Can you work these out from the model? Positions are in its coordinate system, mm. A direction names the side the tool comes from. Give positions to 0.01 mm unless a question says otherwise; leave off trailing zeros. Loops run counter-clockwise (first coordinate to the right, second up) from the corner with the lowest first, then second, coordinate; pieces in that order, holes last. Notation, with made-up numbers: (-6, 58) - (43, 58) arc R3 cw to (43, 62) - close; hole circle Ø3 at (9.25, 2). An arc over 180 degrees is marked (long way). Answer in a Markdown table with one row per item.
Autodesk Inventor part; units mm, degrees
ref_plane "YZ Plane" through (0, 0, 0) normal (1, 0, 0) x (0, 1, 0)
ref_plane "XZ Plane" through (0, 0, 0) normal (0, 1, 0) x (-1, 0, 0)
ref_plane "XY Plane" through (0, 0, 0) normal (0, 0, 1) x (1, 0, 0)
sketch "スケッチ1" plane through (0, 0, 0) normal (0, 0, 1) x (1, 0, 0)
  line L0 (0, 0) -> (142, 0)
  line L1 (142, 0) -> (142, 80)
  line L2 (142, 80) -> (0, 80)
  line L3 (0, 80) -> (0, 0)
  dimension "d40" = 142
  dimension "d41" = 80
extrude "押し出し1" add sketch "スケッチ1" along normal blind 3.3
hole "穴5" at (4.5, 75.5, 3.3) direction (0, 0, -1) diameter 3.4 end through all
hole "穴6" at (137.5, 75.5, 3.3) direction (0, 0, -1) diameter 3.4 end through all
hole "穴7" at (137.5, 4.5, 3.3) direction (0, 0, -1) diameter 3.4 end through all
hole "穴8" at (4.5, 4.5, 3.3) direction (0, 0, -1) diameter 3.4 end through all
hole "穴9" at (130, 73, 3.3) direction (0, 0, -1) diameter 3.4 end through all
hole "穴10" at (130, 7, 3.3) direction (0, 0, -1) diameter 3.4 end through all
hole "穴13" at (41, 73, 3.3) direction (0, 0, -1) diameter 3.4 end through all
hole "穴14" at (41, 7, 3.3) direction (0, 0, -1) diameter 3.4 end through all
sketch "スケッチ2" plane through (0, 0, 3.3) normal (0, 0, 1) x (1, 0, 0)
  line L0 (7, 60) -> (30, 60)
  line L1 (30, 60) -> (30, 47.8)
  line L2 (30, 47.8) -> (7, 47.8)
  line L3 (7, 47.8) -> (7, 60)
  point P0 (0, 0)
  dimension "d132" = 23
  dimension "d133" = 12.2
extrude "押し出し2" cut sketch "スケッチ2" against normal blind 10
hole "穴15" at (5, 53.9, 3.3) direction (0, 0, -1) diameter 2.4 end through all
hole "穴16" at (32, 53.9, 3.3) direction (0, 0, -1) diameter 2.4 end through all
properties part number "基本板上" material "アルミニウム 5052"
Q1. Imagine slicing it at B-B, the plane z = 1.95. Count the separate pieces of the cut face and the enclosed holes in it, and give its area (3 significant figures).
Checked values:
| item | result |
|---|---|
| separate pieces | 1 |
| enclosed holes | 11 |
| area | 11,000 mm² |
Q2. If we mould it in two halves opening along X, with no side actions, what happens to faces 1 (the face through (142, 39, 2)), 2 (the face through (129.93, 74.7, 1.63)), 3 (the face through (70, 0, 2)), 4 (the face through (0, 41, 2))? For each: released by +X, released by -X, zero draft, split by the parting line, or undercut.
Checked values:
| item | result |
|---|---|
| face 1 | released by +X |
| face 2 | undercut |
| face 3 | zero draft |
| face 4 | released by -X |
Q3. If I drill on line 1 (X direction, y = 73, z = 1.05); line 2 (Y direction, x = 137.5, z = 1.3); line 3 (X direction, y = 75.5, z = 0.8), over which ranges is the centre line in solid material (lowest first)? Write a range as [from, to].
Checked values:
| item | result |
|---|---|
| line 1 | x = [0, 39.3], [42.7, 128.3], [131.7, 142] |
| line 2 | y = [0, 2.8], [6.2, 73.8], [77.2, 80] |
| line 3 | x = [0, 2.8], [6.2, 135.8], [139.2, 142] |
Q4. On a 3-axis mill with a long thin cutter (end or side, diameter ignored), from which of +Z, -Z, +X, -X, +Y, -Y can I reach the whole of each face in a straight line? I mean faces 5 (the face through (19, 47.8, 2)), 6 (the face through (70, 41, 3.3)). Say none if no direction works.
Checked values:
| item | result |
|---|---|
| face 5 | +Z, -Z |
| face 6 | +Z, +X, -X, +Y, -Y |
Q5. Imagine slicing it at A-A, the plane x = 137.5. Write out the boundary of the cut face in (y, z).
Checked values:
| item | result |
|---|---|
| outline | (0, 0) - (2.8, 0) - (2.8, 3.3) - (0, 3.3) - close; (6.2, 0) - (73.8, 0) - (73.8, 3.3) - (6.2, 3.3) - close; (77.2, 0) - (80, 0) - (80, 3.3) - (77.2, 3.3) - close |
